```python
from build123d import *

# Parameters (mm, degrees)
F0_W     = 80
F0_H     = 60
F1_DEPTH = 5
F2_R     = 25
F3_DEPTH = 50
F5_DEPTH = 50


with BuildPart() as f1:
    # F0 (on Front) → F1 (new body)
    with BuildSketch(Plane.XZ):
        Rectangle(F0_W, F0_H)
    extrude(amount=F1_DEPTH)

    # F2 (on face) → F3 (join)
    with BuildSketch(Plane.XZ.offset(5)):
        Circle(F2_R)
    extrude(amount=F3_DEPTH)

    # F4 (on face) → F5 (cut)
    with BuildSketch(Plane.XZ.offset(55)):
        Polygon((10.68098, -18.5), (21.36196, 0), (10.68098, 18.5), (-10.68098, 18.5), (-21.36196, 0), (-10.68098, -18.5), align=None)
    extrude(amount=-F5_DEPTH, mode=Mode.SUBTRACT)


solid = f1.part
```
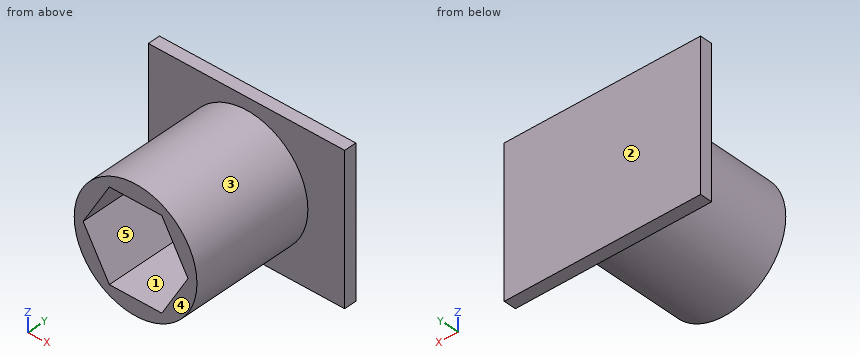
The listing builds one solid part. Answer for the finished solid, in the listing's coordinates (mm). Face numbers are marked on the shaded views. A direction names the side the tool comes from. Coordinates: 2 decimals unless noted, no trailing zeros. Write each loop counter-clockwise with the first axis right and the second up, starting at its lowest first coordinate (ties: lowest second). Pieces come first, ordered by that corner, then holes.
Q1. Section A-A, the plane y = -45 is taken. Write down the section's boundary in (x, z), then the cut area to 3 significant figures.
Returned:
outline: circle Ø50 at (0, 0); hole (-21.36, 0) - (-10.68, -18.5) - (10.68, -18.5) - (21.36, 0) - (10.68, 18.5) - (-10.68, 18.5) - close
area: 778 mm2
Q2. Which of the six approach directions +Z, -Z, +X, -X, +Y, -Y give full straight-line access (tool end or side, diameter ignored) to the marked faces 4 and 5?
Returned:
face 4: +Z, -Z, +X, -X, -Y
face 5: -Y
Q3. Find the intervals of material crossed by line 1 along Z through (x, y) = (-0.5, -30.5) (3 decimals); line 2 along Y through (x, z) = (20, -26.5); line 3 along Z through (x, y) = (-5, -31), in increasing order.
Returned:
line 1: z = -24.995 to -18.5, 18.5 to 24.995
line 2: y = -5 to 0
line 3: z = -24.49 to -18.5, 18.5 to 24.49
Q4. Section B-B, the plane x = 0 is taken. Write down the section's boundary in (y, z), then the cut area to 3 significant figures.
Returned:
outline: (-55, -25) - (-5, -25) - (-5, -30) - (0, -30) - (0, 30) - (-5, 30) - (-5, 25) - (-55, 25) - (-55, 18.5) - (-5, 18.5) - (-5, -18.5) - (-55, -18.5) - close
area: 950 mm2
Q5. Section D-D, the plane x = -14 is taken. Write down the section's boundary in (y, z).
Returned:
outline: (-55, -20.71) - (-5, -20.71) - (-5, -30) - (0, -30) - (0, 30) - (-5, 30) - (-5, 20.71) - (-55, 20.71) - (-55, 12.75) - (-5, 12.75) - (-5, -12.75) - (-55, -12.75) - close
Q6. Given P1, Ø4, axis at y = -23.5, z = -3.5, coming from the -X side; P2, Ø18.5, axis at x = -8.5, z = 1, coming from the -Y side; P3, Ø1.5, axis at y = -34.5, z = -17.5, coming from the +X side; P4, Ø3, axis at x = 18, z = -14.5, coming from the +Y side, each flat-ended and moving along its own axis, determine where each tip first touches the part or whether it passes through.
Returned:
P1: stops at x = -24.95
P2: stops at y = -5
P3: stops at x = 18.56
P4: stops at y = 0
Q7. Section C-C, the plane x = 30 is taken. Write down the section's boundary in (y, z).
Returned:
outline: (-5, -30) - (0, -30) - (0, 30) - (-5, 30) - close
Q8. The mould has two halves that part along Z. Classify the marked faces 1, 2 and 3: released by +Z, released by -Z, zero draft, split by the parting line, or undercut.
Returned:
face 1: undercut
face 2: zero draft
face 3: split by the parting line
